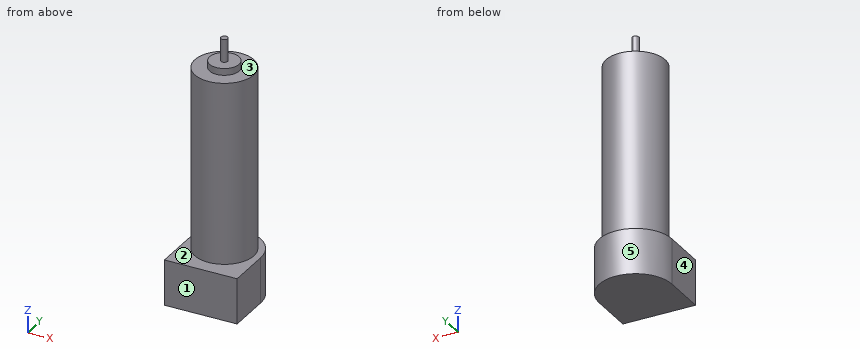
from build123d import *

# Parameters (mm, degrees)
ESQUISSE1_R      = 13
EXTRUSION1_DEPTH = 80
ESQUISSE2_R      = 6.5
EXTRUSION2_DEPTH = 3
ESQUISSE3_R      = 1.5
EXTRUSION3_DEPTH = 10
EXTRUSION5_DEPTH = 20


with BuildPart() as part:
    # Esquisse1 → Extrusion1 (new body)
    with BuildSketch(Plane.XY):
        Circle(ESQUISSE1_R)
    extrude(amount=EXTRUSION1_DEPTH)

    # Esquisse2 → Extrusion2 (add)
    with BuildSketch(Plane.XY.offset(80)):
        Circle(ESQUISSE2_R)
    extrude(amount=EXTRUSION2_DEPTH)

    # Esquisse3 → Extrusion3 (add)
    with BuildSketch(Plane.XY.offset(83)):
        Circle(ESQUISSE3_R)
    extrude(amount=EXTRUSION3_DEPTH)

    # Esquisse4 → Extrusion5 (add)
    with BuildSketch(Plane(origin=(0, 0, 0), x_dir=(-1, 0, 0), z_dir=(0, 0, -1))):
        with BuildLine():
            Line((-16, 0), (-16, -19.313261222))
            Line((-16, -19.313261222), (16, -19.313261222))
            Line((16, -19.313261222), (16, 0))
            ThreePointArc((16, 0), (0, 16), (-16, 0))
        make_face()
    extrude(amount=EXTRUSION5_DEPTH)


solid = part.part
Input: part model. Units: mm. Frame: model coordinates. Face numbers are marked on the shaded views. A direction names the side the tool comes from. Coordinates: 2 decimals unless noted, no trailing zeros. Loops run counter-clockwise (first coordinate to the right, second up) from the corner with the lowest first, then second, coordinate; pieces in that order, holes last.
(1) Section A-A on x = 0. Return the cut outline in (y, z).
(2) Pull-direction query (X, two-part tool) for the marked faces 3, 4 and 5; classes: released by +X, released by -X, zero draft, split by the parting line, or undercut.
(3) First-contact query: pin 1 Ø5 at (x, y) = (6.5, -5) entering from +Z; pin 2 Ø5 at (x, z) = (-9, -7) entering from +Y; pin 3 Ø12 at (y, z) = (10, 38.5) entering from -X. Flat tips, straight axial feed; report the tip coordinate or a pass-through.
(4) Material intervals for probe 1 along Z at (x, y) = (-5.5, 9.5); probe 2 along Z at (x, y) = (-12.5, -9); probe 3 along X at (y, z) = (11, 70.5), sorted ascending.
(5) Section B-B on z = 85.5. Return the cut outline in (x, y), then the cut area to 3 significant figures.
(6) Section D-D on x = 8. Return the cut outline in (y, z), then the cut area to 3 significant figures.
(7) Set-up query: the marked faces 1 and 2. Return all of +Z, -Z, +X, -X, +Y, -Y with unobstructed straight access to the full face (end or side cutting, diameter ignored); none if empty.
(8) Section C-C on y = -17. Return the cut outline in (x, z).
Data:
1. outline: (-19.31, -20) - (16, -20) - (16, 0) - (13, 0) - (13, 80) - (6.5, 80) - (6.5, 83) - (1.5, 83) - (1.5, 93) - (-1.5, 93) - (-1.5, 83) - (-6.5, 83) - (-6.5, 80) - (-13, 80) - (-13, 0) - (-19.31, 0) - close
2. face 3: zero draft
2. face 4: released by -X
2. face 5: split by the parting line
3. pin 1: stops at z = 83
3. pin 2: stops at y = 14.62
3. pin 3: stops at x = -12.37
4. probe 1: z = -20 to 80
4. probe 2: z = -20 to 0
4. probe 3: x = -6.93 to 6.93
5. outline: circle Ø3 at (0, 0)
5. area: 7.07 mm2
6. outline: (-19.31, -20) - (13.86, -20) - (13.86, 0) - (10.25, 0) - (10.25, 80) - (-10.25, 80) - (-10.25, 0) - (-19.31, 0) - close
6. area: 2,300 mm2
7. face 1: +Z, -Z, +X, -X, -Y
7. face 2: +Z
8. outline: (-16, -20) - (16, -20) - (16, 0) - (-16, 0) - close
